```python
from build123d import *

# Parameters (mm, degrees)
SKETCH1_R           = 5.5
SKETCH1_R_2         = 1.5
BOSS_EXTRUDE1_DEPTH = 1.585
SKETCH3_R           = 8.025
CUT_EXTRUDE1_DEPTH  = 2


with BuildPart() as part:
    # Sketch1 → Boss-Extrude1 (new body, symmetric)
    with BuildSketch(Plane.XY):
        with BuildLine():
            Line((25.18, -26.5), (-7.946951673, -26.5))
            ThreePointArc((-7.946951673, -26.5), (-10.721406557, -25.948126611), (-13.073475836, -24.376524164))
            Line((-13.073475836, -24.376524164), (-23.731900423, -13.718099577))
            ThreePointArc((-23.731900423, -13.718099577), (-26.047033407, -10.253258212), (-26.86, -6.166199154))
            Line((-26.86, -6.166199154), (-26.86, 6.166199154))
            ThreePointArc((-26.86, 6.166199154), (-26.047033407, 10.253258212), (-23.731900423, 13.718099577))
            Line((-23.731900423, 13.718099577), (-13.073475836, 24.376524164))
            ThreePointArc((-13.073475836, 24.376524164), (-10.721406557, 25.948126611), (-7.946951673, 26.5))
            Line((-7.946951673, 26.5), (25.18, 26.5))
            ThreePointArc((25.18, 26.5), (30.306524164, 24.376524164), (32.43, 19.25))
            Line((32.43, 19.25), (32.43, -19.25))
            ThreePointArc((32.43, -19.25), (30.306524164, -24.376524164), (25.18, -26.5))
        make_face()
        Circle(SKETCH1_R, mode=Mode.SUBTRACT)
        with Locations((0, 21.9)):
            Circle(SKETCH1_R_2, mode=Mode.SUBTRACT)
        with Locations((-21.9, 0)):
            Circle(SKETCH1_R_2, mode=Mode.SUBTRACT)
        with Locations((0, -21.9)):
            Circle(SKETCH1_R_2, mode=Mode.SUBTRACT)
        with BuildLine():
            Line((17, 22.5), (23.81, 22.5))
            ThreePointArc((23.81, 22.5), (26.31, 20), (23.81, 17.5))
            Line((23.81, 17.5), (17, 17.5))
            ThreePointArc((17, 17.5), (14.5, 20), (17, 22.5))
        make_face(mode=Mode.SUBTRACT)
        with BuildLine():
            Line((17, 12.5), (23.81, 12.5))
            ThreePointArc((23.81, 12.5), (26.31, 10), (23.81, 7.5))
            Line((23.81, 7.5), (17, 7.5))
            ThreePointArc((17, 7.5), (14.5, 10), (17, 12.5))
        make_face(mode=Mode.SUBTRACT)
        with BuildLine():
            Line((17, 2.5), (23.81, 2.5))
            ThreePointArc((23.81, 2.5), (26.31, 0), (23.81, -2.5))
            Line((23.81, -2.5), (17, -2.5))
            ThreePointArc((17, -2.5), (14.5, 0), (17, 2.5))
        make_face(mode=Mode.SUBTRACT)
        with BuildLine():
            Line((17, -7.5), (23.81, -7.5))
            ThreePointArc((23.81, -7.5), (26.31, -10), (23.81, -12.5))
            Line((23.81, -12.5), (17, -12.5))
            ThreePointArc((17, -12.5), (14.5, -10), (17, -7.5))
        make_face(mode=Mode.SUBTRACT)
        with BuildLine():
            Line((17, -17.5), (23.81, -17.5))
            ThreePointArc((23.81, -17.5), (26.31, -20), (23.81, -22.5))
            Line((23.81, -22.5), (17, -22.5))
            ThreePointArc((17, -22.5), (14.5, -20), (17, -17.5))
        make_face(mode=Mode.SUBTRACT)
    extrude(amount=BOSS_EXTRUDE1_DEPTH, both=True)

    # Sketch3 → Cut-Extrude1 (cut)
    with BuildSketch(Plane.XY.offset(1.585)):
        Circle(SKETCH3_R)
    extrude(amount=-CUT_EXTRUDE1_DEPTH, mode=Mode.SUBTRACT)


solid = part.part
```
CAD build for the part. Positions are in the model's coordinates, mm. A direction names the side the tool comes from. Coordinates: 2 decimals unless noted, no trailing zeros. Write each loop counter-clockwise with the first axis right and the second up, starting at its lowest first coordinate (ties: lowest second). Pieces come first, ordered by that corner, then holes. Notation, with made-up numbers: (-16.5, 52.5) -> (34.5, 52.5) arc R20 ccw to (34.5, 69.5) -> close; hole circle Ø1 at (-27, 85.25). An arc over 180 degrees is marked (long way). Return JSON: item names as keys, results as strings. Group by question number.
Q1. Cut at D-D, the plane y = -9. Give the cut face in (x, z) (3 decimals).
Q2. Pull direction X, two halves, no side cores. Call faces 4 (the face through (-26.024, -10.307, 0.022)), 5 (the face through (26.31, 10.05, 0.02)), 6 (the face through (10, 0, 1.585)): released by +X, released by -X, zero draft, split by the parting line, or undercut.
Q3. Cut at C-C, the plane x = -21.9. Give the cut face in (y, z) (3 decimals), then the cut area to 3 significant figures.
Q4. Cut at B-B, the plane x = 19. Give the cut face in (y, z) (3 decimals), then the cut area to 3 significant figures.
Q5. Drill centre lines: line 1 (Y direction, x = 0, z = 0.15) (3 decimals); line 2 (Y direction, x = 24, z = 1.05); line 3 (Y direction, x = 0, z = -0.75). Where is each one in solid material? Low to high.
Q6. Cut at A-A, the plane y = 0. Give the cut face in (x, z) (3 decimals), then the cut area to 3 significant figures.
Q7. Flat gauge pins, fed straight in: pin 1 (1.5 mm diameter, centred on y = 15.5, z = 0.5, fed in from -X); pin 2 (2.5 mm diameter, centred on x = 0, y = -21.9, fed in from -Z). Where does each tip first touch, or does it go through?
Q8. Which spindle directions (+Z, -Z, +X, -X, +Y, -Y) get a long thin tool onto all of the face, cutting with end or side? Do faces 1 (the face through (20, -12.5, 0)), 2 (the face through (-26.86, 0, 0)), 3 (the face through (-6.37, -4.88, 0.6)). Say none if no direction does.
Returned:
{
 "1": {"outline": "(-26.477, -1.585) -> (14.709, -1.585) -> (14.709, 1.585) -> (-26.477, 1.585) -> close; (26.101, -1.585) -> (32.43, -1.585) -> (32.43, 1.585) -> (26.101, 1.585) -> close"},
 "2": {"face 4": "released by -X", "face 5": "undercut", "face 6": "zero draft"},
 "3": {"outline": "(-15.55, -1.585) -> (-1.5, -1.585) -> (-1.5, 1.585) -> (-15.55, 1.585) -> close; (1.5, -1.585) -> (15.55, -1.585) -> (15.55, 1.585) -> (1.5, 1.585) -> close", "area": "89.1 mm2"},
 "4": {"outline": "(-26.5, -1.585) -> (-22.5, -1.585) -> (-22.5, 1.585) -> (-26.5, 1.585) -> close; (-17.5, -1.585) -> (-12.5, -1.585) -> (-12.5, 1.585) -> (-17.5, 1.585) -> close; (-7.5, -1.585) -> (-2.5, -1.585) -> (-2.5, 1.585) -> (-7.5, 1.585) -> close; (2.5, -1.585) -> (7.5, -1.585) -> (7.5, 1.585) -> (2.5, 1.585) -> close; (12.5, -1.585) -> (17.5, -1.585) -> (17.5, 1.585) -> (12.5, 1.585) -> close; (22.5, -1.585) -> (26.5, -1.585) -> (26.5, 1.585) -> (22.5, 1.585) -> close", "area": "88.8 mm2"},
 "5": {"line 1": "y = -26.5 to -23.4, -20.4 to -8.025, 8.025 to 20.4, 23.4 to 26.5", "line 2": "y = -26.5 to -22.49, -17.51 to -12.49, -7.51 to -2.49, 2.49 to 7.51, 12.49 to 17.51, 22.49 to 26.5", "line 3": "y = -26.5 to -23.4, -20.4 to -5.5, 5.5 to 20.4, 23.4 to 26.5"},
 "6": {"outline": "(-26.86, -1.585) -> (-23.4, -1.585) -> (-23.4, 1.585) -> (-26.86, 1.585) -> close; (-20.4, -1.585) -> (-5.5, -1.585) -> (-5.5, -0.415) -> (-8.025, -0.415) -> (-8.025, 1.585) -> (-20.4, 1.585) -> close; (5.5, -1.585) -> (14.5, -1.585) -> (14.5, 1.585) -> (8.025, 1.585) -> (8.025, -0.415) -> (5.5, -0.415) -> close; (26.31, -1.585) -> (32.43, -1.585) -> (32.43, 1.585) -> (26.31, 1.585) -> close", "area": "96.0 mm2"},
 "7": {"pin 1": "stops at x = -22.7", "pin 2": "passes through"},
 "8": {"face 1": "+Z, -Z", "face 2": "+Z, -Z, -X, +Y, -Y", "face 3": "+Z"}
}
